from build123d import *
from build123d.topology import SkipClean

# Parameters (mm, degrees)
BASPROSKE_W         = 12
BASPROSKE_H         = 10.5
TOOTHCUT_DEPTH      = 20.091883092
TEETHCUTS_COUNT     = 19
BORSKE_R            = 2.5
BORE_DEPTH          = 50.0000508
SKETCH1_R           = 5
CUT_EXTRUDE1_DEPTH  = 3
BOSS_EXTRUDE1_DEPTH = 9
SKETCH3_R           = 10.5
SKETCH3_R_2         = 8.249
CUT_EXTRUDE2_DEPTH  = 2
SKETCH4_R           = 8.249
CUT_EXTRUDE3_DEPTH  = 2
BOSS_EXTRUDE3_START = -7
SKETCH5_R           = 2.5
BOSS_EXTRUDE3_DEPTH = 7


with BuildPart() as part:
    # BasProSke → Base-Revolve (revolve)
    with BuildSketch(Plane(origin=(0, 0, 0), x_dir=(1, 0, 0), z_dir=(0, 1, 0)), mode=Mode.PRIVATE) as base_revolve_sk:
        with Locations((6, 5.25)):
            Rectangle(BASPROSKE_W, BASPROSKE_H)
    revolve(base_revolve_sk.sketch.rotate(Axis((-10, 0, 0), (1, 0, 0)), 180), axis=Axis((-10, 0, 0), (1, 0, 0)))

    # TooCutSke → ToothCut (cut, through all)
    with BuildSketch(Plane(origin=(0, 0, 0), x_dir=(0, 0, -1), z_dir=(1, 0, 0))):
        with BuildLine():
            ThreePointArc((0.505024765, 8.233526036), (0, 8.249), (-0.505024765, 8.233526036))
            ThreePointArc((-0.505024765, 8.233526036), (-0.825185426, 9.406360648), (-1.499357972, 10.41805984))
            ThreePointArc((-1.499357972, 10.41805984), (0, 10.5254), (1.499357972, 10.41805984))
            ThreePointArc((1.499357972, 10.41805984), (0.825185426, 9.406360648), (0.505024765, 8.233526036))
        make_face()
    toothcut = extrude(amount=TOOTHCUT_DEPTH, mode=Mode.SUBTRACT)

    # TeethCuts: ToothCut ×19 about axis
    teethcuts_axis = Axis((0, 0, 0), (1, 0, 0))
    for i in range(1, TEETHCUTS_COUNT):
        add(toothcut.rotate(teethcuts_axis, i * 360 / TEETHCUTS_COUNT), mode=Mode.SUBTRACT)

    # BorSke → Bore (cut, symmetric)
    with BuildSketch(Plane(origin=(0, 0, 0), x_dir=(0, 0, -1), z_dir=(1, 0, 0))):
        with Locations(Location((0, 0, 0), (0, 0, 180))):
            Circle(BORSKE_R)
    extrude(amount=BORE_DEPTH, both=True, mode=Mode.SUBTRACT)

    # Sketch1 → Cut-Extrude1 (cut)
    with BuildSketch(Plane(origin=(12, 0, 0), x_dir=(0, 0, -1), z_dir=(1, 0, 0))):
        Circle(SKETCH1_R)
    extrude(amount=-CUT_EXTRUDE1_DEPTH, mode=Mode.SUBTRACT)

    # Sketch2 → Boss-Extrude1 (add)
    with BuildSketch(Plane(origin=(9, 0, 0), x_dir=(0, 0, -1), z_dir=(1, 0, 0))):
        with BuildLine():
            Line((-2.085372664, -1.378847653), (-2.085372664, 1.378847653))
            ThreePointArc((-2.085372664, 1.378847653), (-2.5, 0), (-2.085372664, -1.378847653))
        make_face()
    extrude(amount=-BOSS_EXTRUDE1_DEPTH)

    # Sketch3 → Cut-Extrude2 (cut)
    with SkipClean():  # the faces are left unmerged after this step: merging them gives an invalid solid
        with BuildSketch(Plane.ZY):
            Circle(SKETCH3_R)
            with Locations(Location((0, 0, 0), (0, 0, 358.773146294))):
                Circle(SKETCH3_R_2, mode=Mode.SUBTRACT)
        extrude(amount=-CUT_EXTRUDE2_DEPTH, mode=Mode.SUBTRACT)

    # Sketch4 → Cut-Extrude3 (cut)
    with BuildSketch(Plane.ZY):
        Circle(SKETCH4_R)
    extrude(amount=-CUT_EXTRUDE3_DEPTH, mode=Mode.SUBTRACT)

    # Sketch5 → Boss-Extrude3 (add)
    with BuildSketch(Plane.ZY.offset(-2).offset(BOSS_EXTRUDE3_START)):
        Circle(SKETCH5_R)
    extrude(amount=BOSS_EXTRUDE3_DEPTH)


solid = part.part
Work out the finished part from the listing and answer in its coordinate system (mm). A direction names the side the tool comes from. Give positions to 0.01 mm unless a question says otherwise; leave off trailing zeros. Loops run counter-clockwise (first coordinate to the right, second up) from the corner with the lowest first, then second, coordinate; pieces in that order, holes last. Notation, with made-up numbers: (-15, -12) - (36, -12) arc R24 ccw to (36, 22) - close; hole circle Ø11 at (78.25, -31.5). An arc over 180 degrees is marked (long way). Answer in a Markdown table with one row per item. Add a question column.
Q1. The part is cut by section A-A (z = 0). Determine the outline of the cut face in (x, y), and give its area (3 significant figures).
Q2. Consider line 1 along Y through (x, z) = (11.2, 0); line 2 along Z through (x, y) = (5, 9.25); line 3 along Z through (x, y) = (11, 9). Determine where each line is inside the solid, lowest interval first.
Q3. Determine the mould class of faces 1 (the cylindrical face through (6.93, -8.138, -1.351)), 2 (the flat face through (2, 0, 0)), 3 (the cylindrical face through (6.93, 1.51, -9.32)), 4 (the cylindrical face through (6.93, 0.046, 9.444)) for opening direction Z: released by +Z, released by -Z, zero draft, split by the parting line, or undercut.
Q4. A tool of negligible diameter and unlimited length cuts with its end or side. For faces 5 (the cylindrical face through (6.93, -7.251, 3.932)), 6 (the cylindrical face through (6.93, -1.6, -9.31)), 7 (the cylindrical face through (6.93, -9.14, 2.36)), from which of +Z, -Z, +X, -X, +Y, -Y can it reach the whole face along a straight path? Write none if from no direction.
Q5. Each of these flat-tipped pins is pushed along its axis until it touches: P1, Ø5, axis at x = 5.5, y = 5.5, coming from the +Z side; P2, Ø5, axis at x = 5, z = 8.5, coming from the +Y side; P3, Ø5, axis at x = 10, y = -3, coming from the -Z side. Where does it stop, or does it pass through?
Solution:
| question | item | result |
|---|---|---|
| 1 | outline | (2, -10.5) - (12, -10.5) - (12, -5) - (9, -5) - (9, 5) - (12, 5) - (12, 8.25) - (2, 8.25) - close |
| 1 | area | 157 mm² |
| 2 | line 1 | y = -10.5 to -5, 5 to 8.25 |
| 2 | line 2 | z = -4.97 to -4.6, -2.26 to -0.76, 0.76 to 2.26, 4.6 to 4.97 |
| 2 | line 3 | z = -5.23 to -4.24, -2.29 to -0.67, 0.67 to 2.29, 4.24 to 5.23 |
| 3 | face 1 | undercut |
| 3 | face 2 | zero draft |
| 3 | face 3 | undercut |
| 3 | face 4 | released by +Z |
| 4 | face 5 | +X, -X |
| 4 | face 6 | -Z, +X, -X |
| 4 | face 7 | +X, -X, -Y |
| 5 | P1 | stops at z = 9.71 |
| 5 | P2 | stops at y = 7.3 |
| 5 | P3 | stops at z = -10.24 |
